```python
from build123d import *

# Parameters (mm, degrees)
EXTRUDE_1_DEPTH = 4


with BuildPart() as part:
    # Эскиз1 → Бобышка-Вытянуть1 (new body)
    with BuildSketch(Plane(origin=(0, 0, 0), x_dir=(1, 0, 0), z_dir=(0, 1, 0))):
        Polygon((0, 0), (0, -14), (3.103725277, -14), (15, -8.452675993), (15, 0), align=None)
    extrude(amount=EXTRUDE_1_DEPTH)

    # Эскиз2 → Цековка для  винта с внутренним шестигранником #41 (revolve, cut)
    with BuildSketch(Plane(origin=(3.5, 4, 9.5), x_dir=(0, 0, 1), z_dir=(1, 0, 0))):
        Polygon((0, 0), (0, 4), (1.6002, 4), (1.4732, 3.873), (1.4732, 2.9718), (1.6002, 2.8448), (2.77876, 2.8448), (2.77876, 0), align=None)
    revolve(axis=Axis((3.5, 10.35, 9.5), (0, -1, 0)), mode=Mode.SUBTRACT)


solid = part.part
```
For this review, take the finished solid that the model builds, in its own axes (mm). A direction names the side the tool comes from. Round coordinates to 2 decimals unless told otherwise and drop trailing zeros. Loops run counter-clockwise (first coordinate to the right, second up) from the corner with the lowest first, then second, coordinate; pieces in that order, holes last.
(1) We need section B-B (y = 0.35). Give the boundary of the cut face in (x, z).
Returned:
outline: (0, 0) - (15, 0) - (15, 8.45) - (3.1, 14) - (0, 14) - close; hole circle Ø2.95 at (3.5, 9.5)
(2) Wall thickness on line 1 along X through (y, z) = (2.25, 10.25); line 2 along X through (y, z) = (2.85, 9.5); line 3 along Z through (x, y) = (3.5, 0.6): over which ranges is each line inside the solid? List them lowest first.
Returned:
line 1: x = 0 to 0.82, 6.18 to 11.15
line 2: x = 0 to 0.72, 6.28 to 12.75
line 3: z = 0 to 8.03, 10.97 to 13.82
(3) We need section C-C (x = 3.5). Give the boundary of the cut face in (y, z).
Returned:
outline: (0, 0) - (4, 0) - (4, 6.72) - (1.16, 6.72) - (1.16, 7.9) - (1.03, 8.03) - (0.13, 8.03) - (0, 7.9) - close; (0, 11.1) - (0.13, 10.97) - (1.03, 10.97) - (1.16, 11.1) - (1.16, 12.28) - (4, 12.28) - (4, 13.82) - (0, 13.82) - close
(4) We need section A-A (z = 9.5). Give the boundary of the cut face in (x, y), plus the area to 3 significant figures.
Returned:
outline: (0, 0) - (1.9, 0) - (2.03, 0.13) - (2.03, 1.03) - (1.9, 1.16) - (0.72, 1.16) - (0.72, 4) - (0, 4) - close; (4.97, 0.13) - (5.1, 0) - (12.75, 0) - (12.75, 4) - (6.28, 4) - (6.28, 1.16) - (5.1, 1.16) - (4.97, 1.03) - close
area: 31.8 mm2
(5) We need section D-D (x = 1.5). Give the boundary of the cut face in (y, z).
Returned:
outline: (0, 0) - (4, 0) - (4, 7.57) - (1.16, 7.57) - (1.16, 11.43) - (4, 11.43) - (4, 14) - (0, 14) - close
(6) Mouldability with a two-part tool opening along Z and no side actions: class faces 1 (the flat face through (0, 2, 7)), 2 (the flat face through (8.969, 1.972, 11.265)), 3 (the flat face through (5, 1.155, 8)) as released by +Z, released by -Z, zero draft, split by the parting line, or undercut.
Returned:
face 1: zero draft
face 2: released by +Z
face 3: undercut
(7) Tool access review of faces 4 (the flat face through (15, 2, 4)), 5 (the cylindrical face through (4.56, 2.6, 12.07)): name each direction out of +Z, -Z, +X, -X, +Y, -Y from which nothing blocks a thin tool from reaching the whole face with its end or side.
Returned:
face 4: +Z, -Z, +X, +Y, -Y
face 5: +Y
